Can you work these out from the model? Positions are in its coordinate system, mm. Face numbers are marked on the shaded views. A direction names the side the tool comes from. Give positions to 0.01 mm unless a question says otherwise; leave off trailing zeros. Loops run counter-clockwise (first coordinate to the right, second up) from the corner with the lowest first, then second, coordinate; pieces in that order, holes last.
from build123d import *

# Parameters (mm, degrees)
ESQUISSE1_W             = 200
ESQUISSE1_H             = 30
ESQUISSE1_R             = 2.5
BOSS_EXTRU_1_DEPTH      = 3
ESQUISSE2_W             = 3
ESQUISSE2_H             = 30
BOSS_EXTRU_2_DEPTH      = 25
ESQUISSE3_R             = 3
ENL_V_MAT_EXTRU_1_DEPTH = 229
CONG_1_R                = 2


with BuildPart() as part:
    # Esquisse1 → Boss.-Extru.1 (new body)
    with BuildSketch(Plane.XY):
        with Locations((100, -15)):
            Rectangle(ESQUISSE1_W, ESQUISSE1_H)
        with Locations((40, -15)):
            Circle(ESQUISSE1_R, mode=Mode.SUBTRACT)
        with Locations((160, -15)):
            Circle(ESQUISSE1_R, mode=Mode.SUBTRACT)
    extrude(amount=BOSS_EXTRU_1_DEPTH)

    # Esquisse2 → Boss.-Extru.2 (add)
    with BuildSketch(Plane.XY.offset(3)):
        with Locations((1.5, -15)):
            Rectangle(ESQUISSE2_W, ESQUISSE2_H)
        with Locations((198.5, -15)):
            Rectangle(ESQUISSE2_W, ESQUISSE2_H)
    extrude(amount=BOSS_EXTRU_2_DEPTH)

    # Esquisse3 → Enlèv. mat.-Extru.1 (cut)
    with BuildSketch(Plane.ZY):
        with Locations((15, -15)):
            Circle(ESQUISSE3_R)
    extrude(amount=-ENL_V_MAT_EXTRU_1_DEPTH, mode=Mode.SUBTRACT)

    # Congé1
    cong_1_edges = [part.edges().sort_by_distance(p)[0] for p in [
        (3, -15, 3),
        (197, -15, 3),
        (200, -15, 0),
        (0, -15, 0),
    ]]
    fillet(cong_1_edges, radius=CONG_1_R)


solid = part.part
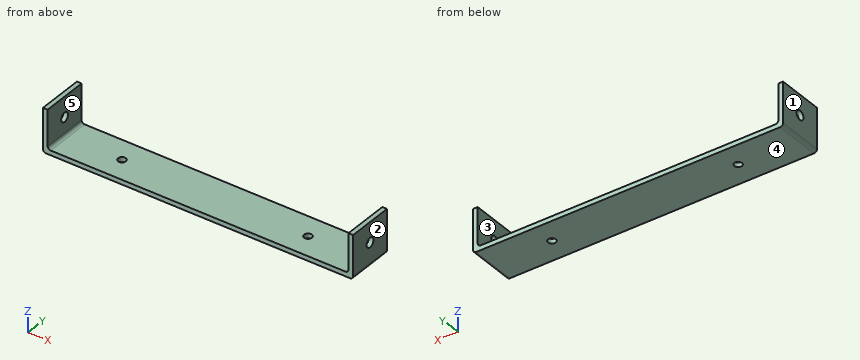
(1) Which directions (+Z, -Z, +X, -X, +Y, -Y) give clear straight access to the entire face, cutting with the end or side of a thin tool? Please do the marked faces 4 and 5.
Returned:
face 4: -Z, +X, -X, +Y, -Y
face 5: +Z, +Y, -Y
(2) Suppose I cut it at A-A on z = 15. List the corners of the cut face in (x, y) for me, plus the area to 3 significant figures.
Returned:
outline: (0, -30) - (3, -30) - (3, -18) - (0, -18) - close; (0, -12) - (3, -12) - (3, 0) - (0, 0) - close; (197, -30) - (200, -30) - (200, -18) - (197, -18) - close; (197, -12) - (200, -12) - (200, 0) - (197, 0) - close
area: 144 mm2
(3) Will these pins go through, and if not, where does the flat tip stop? P1, Ø10, axis at x = 172.5, y = -24, coming from the +Z side; P2, Ø9.5, axis at y = -15, z = 15, coming from the +X side.
Returned:
P1: stops at z = 3
P2: stops at x = 200
(4) Thinking about a two-plate mould opening in X: for the marked faces 1, 2 and 3, which applies, pulls with the +X half, pulls with the -X half, needs draft (parallel to the pull), parting line crosses it, or undercut?
Returned:
face 1: pulls with the -X half
face 2: pulls with the +X half
face 3: undercut
(5) Suppose I cut it at D-D on x = 40. List the corners of the cut face in (y, z) for me.
Returned:
outline: (-30, 0) - (-17.5, 0) - (-17.5, 3) - (-30, 3) - close; (-12.5, 0) - (0, 0) - (0, 3) - (-12.5, 3) - close
(6) Suppose I cut it at C-C on z = 26. List the corners of the cut face in (x, y) for me.
Returned:
outline: (0, -30) - (3, -30) - (3, 0) - (0, 0) - close; (197, -30) - (200, -30) - (200, 0) - (197, 0) - close
(7) Suppose I cut it at B-B on y = -15. List the corners of the cut face in (x, z) for me, plus the area to 3 significant figures.
Returned:
outline: (0, 2) arc R2 ccw to (2, 0) - (37.5, 0) - (37.5, 3) - (5, 3) arc R2 cw to (3, 5) - (3, 12) - (0, 12) - close; (0, 18) - (3, 18) - (3, 28) - (0, 28) - close; (42.5, 0) - (157.5, 0) - (157.5, 3) - (42.5, 3) - close; (162.5, 0) - (198, 0) arc R2 ccw to (200, 2) - (200, 12) - (197, 12) - (197, 5) arc R2 cw to (195, 3) - (162.5, 3) - close; (197, 18) - (200, 18) - (200, 28) - (197, 28) - close
area: 684 mm2
(8) Please list where these lines run through material, in increasing order: probe 1 along X at (y, z) = (-23.75, 4.75); probe 2 along Y at (x, z) = (40, 1.3); probe 3 along Z at (x, y) = (27.5, -21.25).
Returned:
probe 1: x = 0 to 3.02, 196.98 to 200
probe 2: y = -30 to -17.5, -12.5 to 0
probe 3: z = 0 to 3
